Part model, mm, in its own coordinate system. Round coordinates to 2 decimals unless told otherwise and drop trailing zeros. Loops run counter-clockwise (first coordinate to the right, second up) from the corner with the lowest first, then second, coordinate; pieces in that order, holes last.
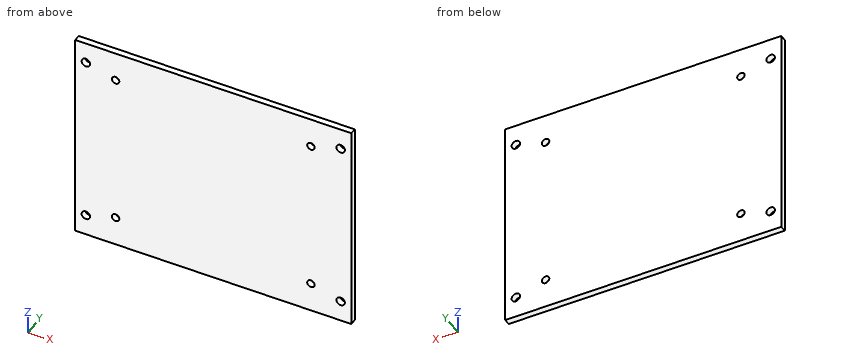
from build123d import *

# Parameters (mm, degrees)
ESBO_O2_W                = 130
ESBO_O2_H                = 100
RESSALTO_EXTRUS_O1_DEPTH = 3
ESBO_O5_R                = 1.75
CORTE_EXTRUS_O1_DEPTH    = 3
ESBO_O6_R                = 2
CORTE_EXTRUS_O2_DEPTH    = 10
ESBO_O7_R                = 2
CORTE_EXTRUS_O3_DEPTH    = 10
ESBO_O8_R                = 2
CORTE_EXTRUS_O4_DEPTH    = 10


with BuildPart() as part:
    # Esboço2 → Ressalto-extrusão1 (new body)
    with BuildSketch(Plane(origin=(0, 0, 0), x_dir=(1, 0, 0), z_dir=(0, 1, 0))):
        with Locations((-65, 50)):
            Rectangle(ESBO_O2_W, ESBO_O2_H)
    extrude(amount=RESSALTO_EXTRUS_O1_DEPTH)

    # Esboço5 → Corte-extrusão1 (cut)
    with BuildSketch(Plane(origin=(0, 3, 0), x_dir=(1, 0, 0), z_dir=(0, 1, 0))):
        with Locations(Location((-111, 86, 0), (0, 0, 270))):
            Circle(ESBO_O5_R)
        with Locations(Location((-19, 86, 0), (0, 0, 270))):
            Circle(ESBO_O5_R)
        with Locations(Location((-19, 14, 0), (0, 0, 270))):
            Circle(ESBO_O5_R)
        with Locations(Location((-111, 14, 0), (0, 0, 270))):
            Circle(ESBO_O5_R)
    extrude(amount=-CORTE_EXTRUS_O1_DEPTH, mode=Mode.SUBTRACT)

    # Esboço6 → Corte-extrusão2 (cut)
    with BuildSketch(Plane(origin=(0, 3, 0), x_dir=(1, 0, 0), z_dir=(0, 1, 0))):
        with Locations(Location((-5, 90, 0), (0, 0, 270))):
            Circle(ESBO_O6_R)
        with Locations(Location((-125, 90, 0), (0, 0, 270))):
            Circle(ESBO_O6_R)
    extrude(amount=-CORTE_EXTRUS_O2_DEPTH, mode=Mode.SUBTRACT)

    # Esboço7 → Corte-extrusão3 (cut)
    with BuildSketch(Plane(origin=(0, 3, 0), x_dir=(1, 0, 0), z_dir=(0, 1, 0))):
        with Locations(Location((-125, 10, 0), (0, 0, 270))):
            Circle(ESBO_O7_R)
    extrude(amount=-CORTE_EXTRUS_O3_DEPTH, mode=Mode.SUBTRACT)

    # Esboço8 → Corte-extrusão4 (cut)
    with BuildSketch(Plane(origin=(0, 3, 0), x_dir=(1, 0, 0), z_dir=(0, 1, 0))):
        with Locations(Location((-5, 10, 0), (0, 0, 270))):
            Circle(ESBO_O8_R)
    extrude(amount=-CORTE_EXTRUS_O4_DEPTH, mode=Mode.SUBTRACT)


solid = part.part
1) Slice it at B-B, the plane x = -111. Give the cut face in (y, z).
Values:
outline: (0, -100) - (3, -100) - (3, -87.75) - (0, -87.75) - close; (0, -84.25) - (3, -84.25) - (3, -15.75) - (0, -15.75) - close; (0, -12.25) - (3, -12.25) - (3, 0) - (0, 0) - close
2) Drop a flat-ended pin along its axis: pin 1 Ø2 at (x, z) = (-111, -14) entering from +Y. Give the stop position or say it passes through.
Values:
pin 1: passes through
3) Slice it at A-A, the plane z = -90. Give the cut face in (x, y).
Values:
outline: (-130, 0) - (-127, 0) - (-127, 3) - (-130, 3) - close; (-123, 0) - (-7, 0) - (-7, 3) - (-123, 3) - close; (-3, 0) - (0, 0) - (0, 3) - (-3, 3) - close
4) Wall check: line 1 along X through (y, z) = (1.5, -90); line 2 along X through (y, z) = (2.35, -86); line 3 along Z through (x, y) = (-112, 2.7). Give the ranges that are in metal, low to high.
Values:
line 1: x = -130 to -127, -123 to -7, -3 to 0
line 2: x = -130 to -112.75, -109.25 to -20.75, -17.25 to 0
line 3: z = -100 to -87.44, -84.56 to -15.44, -12.56 to 0
